The listing builds one solid part. Answer for the finished solid, in the listing's coordinates (mm). Face numbers are marked on the shaded views. Round coordinates to 2 decimals unless told otherwise and drop trailing zeros. Order: outer loops, then holes, each group sorted by start corner. A loop starts at its lowest first (then second) coordinate and runs counter-clockwise, first axis right, second up. Notation, with made-up numbers: M 21.5,-15 L 68.5,-15 A23 cw 68.5,9 Z; hole C 75.25,17 d6. An arc over 180 degrees is marked long. Write item = value, one per line. Start each with the question number.
(1) A cutting plane is placed at C-C, the plane z = -14.5. Determine the outline of the cut face in (x, y).
(2) For a pull along Z with two mould halves and no side action, classify the marked faces 1, 2 and 3 as released by +Z, released by -Z, zero draft, split by the parting line, or undercut.
(3) A cutting plane is placed at B-B, the plane z = -42. Determine the outline of the cut face in (x, y).
(4) A cutting plane is placed at A-A, the plane x = 21.5. Determine the outline of the cut face in (y, z), and give its area (3 significant figures).
(5) Straight lines are drawn through the part: probe 1 along Y at (x, z) = (53, 0); probe 2 along Z at (x, y) = (3, 34.5); probe 3 along Z at (x, y) = (76, -73). For each, find the intervals that lie inside material, in ascending order. Write a range as from..to.
(6) Each of these flat-tipped pins is pushed along its axis until it touches: pin 1 (3 mm diameter, centred on x = 47.5, z = -8.5, fed in from +Y); pin 2 (4 mm diameter, centred on x = 10, z = 44.5, fed in from -Y); pin 3 (3 mm diameter, centred on x = 20.5, y = 51, fed in from -Z). Where does it stop, or does it pass through?
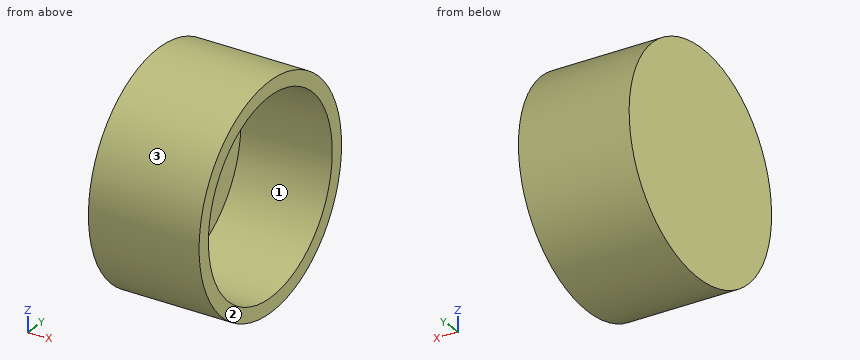
Autodesk Inventor part; units mm, degrees
ref_plane "YZ Plane" through (0, 0, 0) normal (1, 0, 0) x (0, 1, 0)
ref_plane "XZ Plane" through (0, 0, 0) normal (0, 1, 0) x (-1, 0, 0)
ref_plane "XY Plane" through (0, 0, 0) normal (0, 0, 1) x (1, 0, 0)
sketch "Esquisse1" plane through (0, 0, 0) normal (1, 0, 0) x (0, 1, 0)
  circle A0 centre (0, 0) radius 115
  dimension "d0" = 230
extrude "Extrusion1" add sketch "Esquisse1" along normal blind 95
sketch "Esquisse2" plane through (95, 0, 0) normal (1, 0, 0) x (0, 0, -1)
  circle A0 centre (0, 0) radius 100
  dimension "d3" = 200
extrude "Extrusion2" cut sketch "Esquisse2" against normal blind 95
sketch "Esquisse3" plane through (0, 0, 0) normal (-1, 0, 0) x (0, 0, 1)
  circle A0 centre (0, 0) radius 115
  dimension "d6" = 230
extrude "Extrusion3" add sketch "Esquisse3" along normal blind 20
Reported:
q1.outline = M -20,-114.08 L 95,-114.08 L 95,-98.94 L 0,-98.94 L 0,98.94 L 95,98.94 L 95,114.08 L -20,114.08 Z
q2.face_1 = undercut
q2.face_2 = zero draft
q2.face_3 = split by the parting line
q3.outline = M -20,-107.06 L 95,-107.06 L 95,-90.75 L 0,-90.75 L 0,90.75 L 95,90.75 L 95,107.06 L -20,107.06 Z
q4.outline = C 0,0 d230; hole C 0,0 d200
q4.area = 10,100 mm²
q5.probe_1 = -115..-100, 100..115
q5.probe_2 = -109.7..-93.86, 93.86..109.7
q5.probe_3 = -88.86..-68.34, 68.34..88.86
q6.pin_1 = 114.79
q6.pin_2 = -106.86
q6.pin_3 = -103.8
